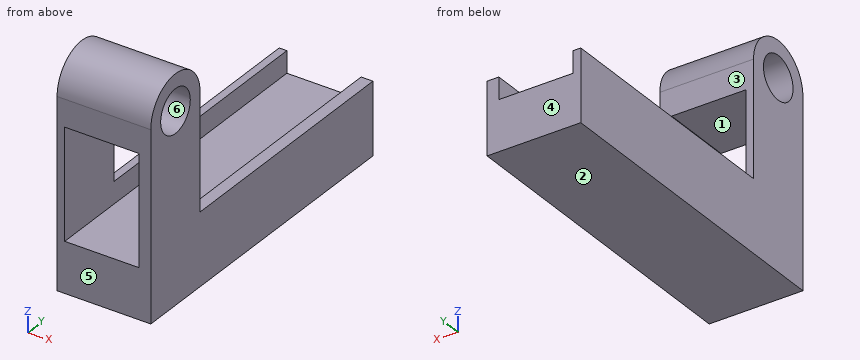
```python
from build123d import *

# Parameters (mm, degrees)
SKETCH_R     = 3
PAD_DEPTH    = 13
SKETCH001_W  = 15.280671
SKETCH001_H  = 10.299273
POCKET_DEPTH = 46


with BuildPart() as part:
    # Sketch → Pad (new body)
    with BuildSketch(Plane.YZ):
        with BuildLine():
            Line((0, 0), (45, 0))
            Line((45, 0), (45, 10))
            Line((45, 10), (20, 10))
            Line((20, 10), (10, 10))
            Line((10, 10), (10, 26))
            ThreePointArc((10, 26), (5, 31), (0, 26))
            Line((0, 26), (0, 0))
        make_face()
        with Locations((5, 26)):
            Circle(SKETCH_R, mode=Mode.SUBTRACT)
    extrude(amount=PAD_DEPTH)

    # Sketch001 (on DatumPlane) → Pocket (cut)
    with BuildSketch(Plane.ZX.offset(45)):
        with Locations((14.617652, 6.211655)):
            Rectangle(SKETCH001_W, SKETCH001_H)
    extrude(amount=-POCKET_DEPTH, mode=Mode.SUBTRACT)


solid = part.part
```
Model file for the job. Use its own axes, mm. Face numbers are marked on the shaded views. A direction names the side the tool comes from. Round coordinates to 2 decimals unless told otherwise and drop trailing zeros. Order: outer loops, then holes, each group sorted by start corner. A loop starts at its lowest first (then second) coordinate and runs counter-clockwise, first axis right, second up. Notation, with made-up numbers: (23.25, -13.75) -> (79.25, -13.75) arc R27 cw to (79.25, 25.25) -> close; hole circle Ø2 at (-3.5, 89.5). An arc over 180 degrees is marked (long way). Use one line per item in the form item = value.
Item 1: Cut at B-B, the plane y = 5. Write the cut outline in (x, z), and give its area (3 significant figures).
Returned:
outline = (0, 0) -> (13, 0) -> (13, 23) -> (0, 23) -> close; (0, 29) -> (13, 29) -> (13, 31) -> (0, 31) -> close; hole (1.06, 6.98) -> (11.36, 6.98) -> (11.36, 22.26) -> (1.06, 22.26) -> close
area = 168 mm^2
Item 2: Cut at D-D, the plane z = 27.5. Write the cut outline in (x, y), and give its area (3 significant figures).
Returned:
outline = (0, 0.23) -> (13, 0.23) -> (13, 2.4) -> (0, 2.4) -> close; (0, 7.6) -> (13, 7.6) -> (13, 9.77) -> (0, 9.77) -> close
area = 56.5 mm^2
Item 3: Flat gauge pins, fed straight in: pin 1 Ø4 at (x, y) = (9.5, 17) entering from +Z; pin 2 Ø6.5 at (x, z) = (3.5, 17) entering from +Y; pin 3 Ø3 at (x, y) = (6.5, 14) entering from +Z. Where does each tip first touch, or does it go through?
Returned:
pin_1 = 10
pin_2 = 10
pin_3 = 6.98
Item 4: Pull direction Y, two halves, no side cores. Call the marked faces 4, 5 and 6: released by +Y, released by -Y, zero draft, split by the parting line, or undercut.
Returned:
face_4 = released by +Y
face_5 = released by -Y
face_6 = undercut
Item 5: Drill centre lines: line 1 (Z direction, x = 3.25, y = 5); line 2 (X direction, y = 5, z = 13.5); line 3 (Z direction, x = 12.75, y = 31). Where is each one in solid material? Low to high.
Returned:
line_1 = 0 to 6.98, 22.26 to 23, 29 to 31
line_2 = 0 to 1.06, 11.36 to 13
line_3 = 0 to 10
Item 6: Cut at C-C, the plane z = 12.5. Write the cut outline in (x, y).
Returned:
outline = (0, 0) -> (1.06, 0) -> (1.06, 10) -> (0, 10) -> close; (11.36, 0) -> (13, 0) -> (13, 10) -> (11.36, 10) -> close
Item 7: Tool access for the marked faces 1, 2 and 3: list every direction of +Z, -Z, +X, -X, +Y, -Y with a clear straight run to the whole face (end or side of a thin tool).
Returned:
face_1 = +Y, -Y
face_2 = -Z, +X, -X, +Y, -Y
face_3 = +Z, +X, -X, +Y
Item 8: Cut at A-A, the plane x = 4.75. Write the cut outline in (y, z).
Returned:
outline = (0, 0) -> (45, 0) -> (45, 6.98) -> (0, 6.98) -> close; (0, 22.26) -> (10, 22.26) -> (10, 26) arc R5 ccw to (0, 26) -> close; hole circle Ø6 at (5, 26)
